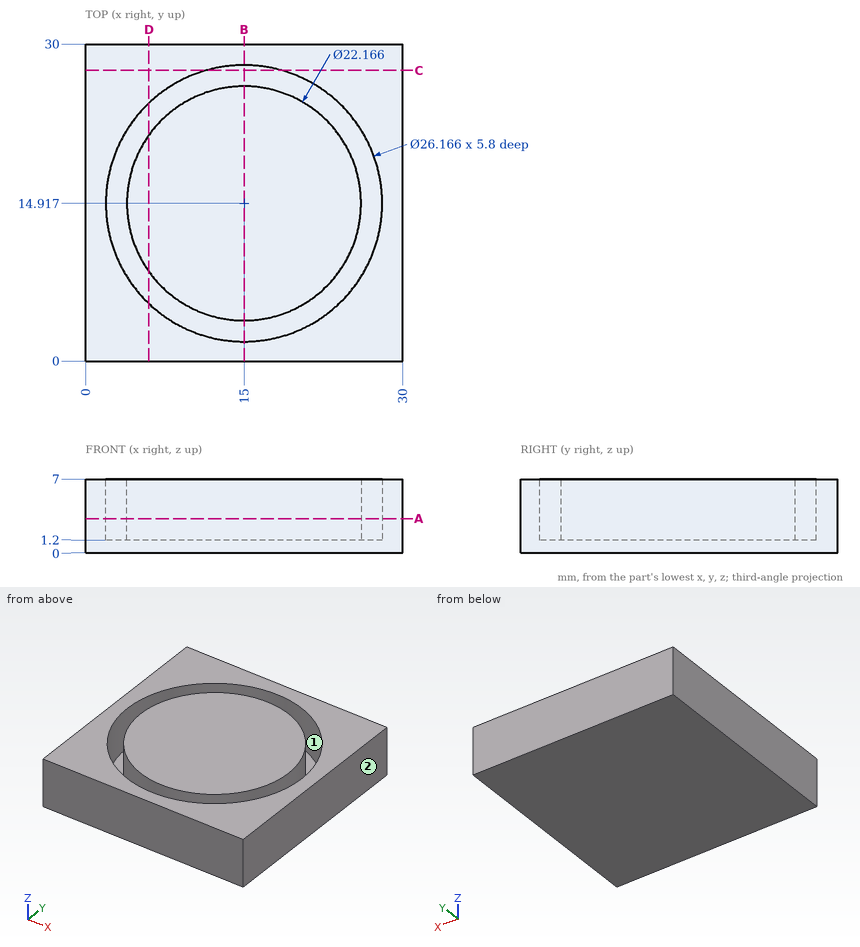
Could you check a few things on this drawing? It's one solid part, dimensions in mm from its lowest x, y, z. A direction names the side the tool comes from. Round coordinates to 2 decimals unless told otherwise and drop trailing zeros. Order: outer loops, then holes, each group sorted by start corner. A loop starts at its lowest first (then second) coordinate and runs counter-clockwise, first axis right, second up. Notation, with made-up numbers: M 33,72.25 L 52,72.25 A9 ccw 52,77.25 Z; hole C 25.25,16 d5. An arc over 180 degrees is marked long. Use a Markdown table: item, result.
1) Imagine slicing it at A-A (z = 3.25). List the corners of the cut face in (x, y) for me, then the cut area to 3 significant figures.
Geometry says:
| item | result |
|---|---|
| outline | M 0,0 L 30,0 L 30,30 L 0,30 Z; C 15,14.92 d22.17; hole C 15,14.92 d26.17 |
| area | 748 mm² |
2) I'm going to push a flat-ended pin straight in: P1, Ø1, axis at x = 17, z = 3.5, coming from the -Y side. Where does the tip first touch, or does it pass through?
Geometry says:
| item | result |
|---|---|
| P1 | stops at y = 0 |
3) Imagine slicing it at C-C (y = 27.5). List the corners of the cut face in (x, z) for me.
Geometry says:
| item | result |
|---|---|
| outline | M 0,0 L 30,0 L 30,7 L 18.58,7 L 18.58,1.2 L 11.42,1.2 L 11.42,7 L 0,7 Z |
4) If I drill on line 1 along Y through (x, z) = (15, 2.6); line 2 along X through (y, z) = (17, 5.5); line 3 along Y through (x, z) = (23, 6), over which ranges is the centre line in solid material (lowest first)?
Geometry says:
| item | result |
|---|---|
| line 1 | y = 0 to 1.83, 3.83 to 26, 28 to 30 |
| line 2 | x = 0 to 2.08, 4.11 to 25.89, 27.92 to 30 |
| line 3 | y = 0 to 4.56, 7.25 to 22.59, 25.27 to 30 |
5) Imagine slicing it at D-D (x = 6). List the corners of the cut face in (y, z) for me, then the cut area to 3 significant figures.
Geometry says:
| item | result |
|---|---|
| outline | M 0,0 L 30,0 L 30,7 L 24.41,7 L 24.41,1.2 L 21.38,1.2 L 21.38,7 L 8.45,7 L 8.45,1.2 L 5.42,1.2 L 5.42,7 L 0,7 Z |
| area | 175 mm² |
6) On a 3-axis mill with a long thin cutter (end or side, diameter ignored), from which of +Z, -Z, +X, -X, +Y, -Y can I reach the whole of each face in a straight line? I mean the marked faces 1 and 2. Say none if no direction works.
Geometry says:
| item | result |
|---|---|
| face 1 | +Z |
| face 2 | +Z, -Z, +X, +Y, -Y |
7) Imagine slicing it at B-B (x = 15). List the corners of the cut face in (y, z) for me, then the cut area to 3 significant figures.
Geometry says:
| item | result |
|---|---|
| outline | M 0,0 L 30,0 L 30,7 L 28,7 L 28,1.2 L 26,1.2 L 26,7 L 3.83,7 L 3.83,1.2 L 1.83,1.2 L 1.83,7 L 0,7 Z |
| area | 187 mm² |
